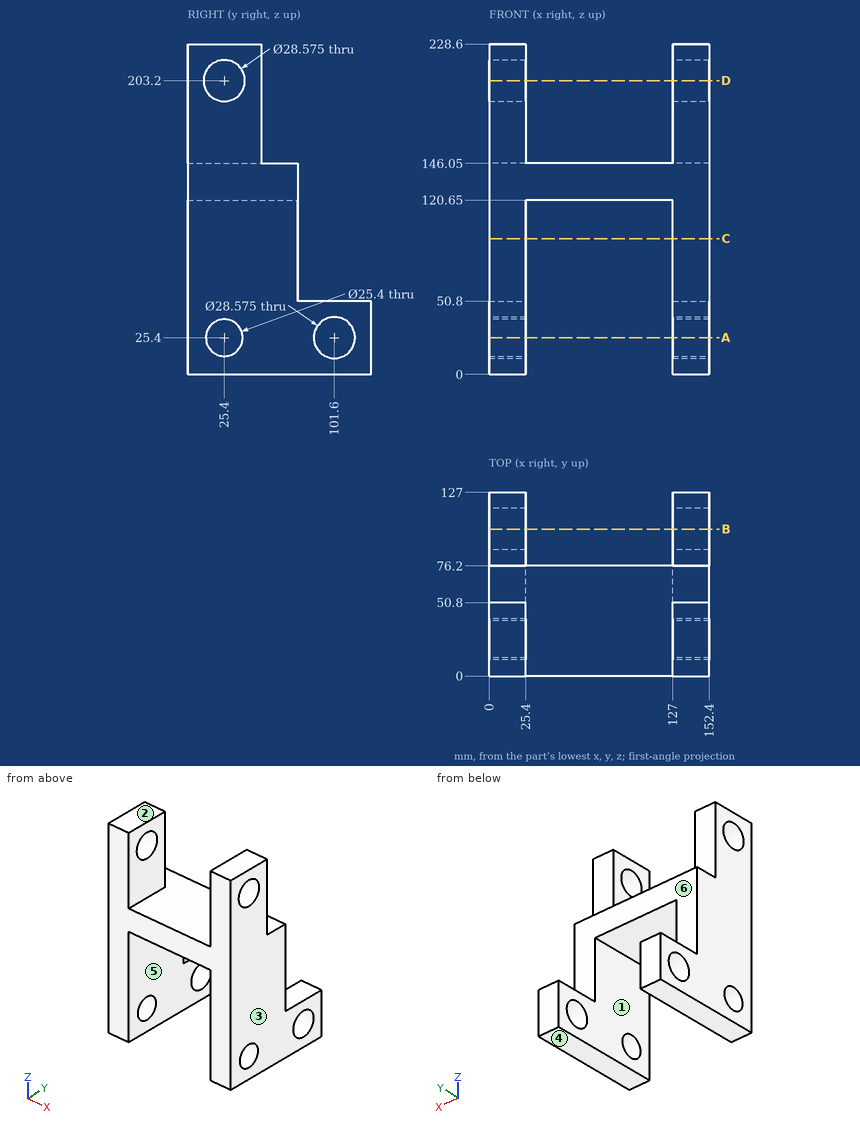
Can you work these out from the drawing? Everything is in mm from the part's minimum corner. A direction names the side the tool comes from. Give positions to 0.01 mm unless a question says otherwise; leave off trailing zeros. Write each loop counter-clockwise with the first axis right and the second up, starting at its lowest first coordinate (ties: lowest second). Pieces come first, ordered by that corner, then holes. Notation, with made-up numbers: M -2.75,-9 L 1.25,-9 A15 cw 1.25,10 Z; hole C 62.5,52 d2. An arc over 180 degrees is marked long. Answer in a Markdown table with one row per item. Add a question column.
Item 1: For pin 1 Ø2 at (x, z) = (24, 62.5) entering from +Y; pin 2 Ø2 at (x, y) = (26, 58) entering from +Z; pin 3 Ø20.5 at (x, z) = (135, 172.5) entering from +Y; pin 4 Ø10 at (x, z) = (42, 151.5) entering from -Y, each with a flat end and sliding along its axis, tell me the tip position at first contact or that it passes through.
Item 2: Imagine slicing it at B-B, the plane y = 101.6. Write out the boundary of the cut face in (x, z).
Item 3: On a 3-axis mill with a long thin cutter (end or side, diameter ignored), from which of +Z, -Z, +X, -X, +Y, -Y can I reach the whole of each face in a straight line? I mean the marked faces 4, 5 and 6. Say none if no direction works.
Item 4: Imagine slicing it at A-A, the plane z = 25.4. Write out the boundary of the cut face in (x, y).
Item 5: We'd pull the mould along X, two halves only. Please class the marked faces 1, 2 and 3: released by +X, released by -X, zero draft, split by the parting line, or undercut.
Item 6: Imagine slicing it at C-C, the plane z = 94. Write out the boundary of the cut face in (x, y), plus the area to 3 significant figures.
Item 7: Please list where these lines run through material, in increasing order: L1, parallel to Y at x = 143, z = 25; L2, parallel to X at y = 66, z = 65; L3, parallel to Z at x = 139, y = 25.
Evaluation:
| question | item | result |
|---|---|---|
| 1 | pin 1 | stops at y = 76.2 |
| 1 | pin 2 | stops at z = 146.05 |
| 1 | pin 3 | stops at y = 50.8 |
| 1 | pin 4 | passes through |
| 2 | outline | M 0,0 L 25.4,0 L 25.4,11.11 L 0,11.11 Z; M 0,39.69 L 25.4,39.69 L 25.4,50.8 L 0,50.8 Z; M 127,0 L 152.4,0 L 152.4,11.11 L 127,11.11 Z; M 127,39.69 L 152.4,39.69 L 152.4,50.8 L 127,50.8 Z |
| 3 | face 4 | -Z, +X, -X, +Y, -Y |
| 3 | face 5 | -Z, +Y, -Y |
| 3 | face 6 | +Z, +X, -X, +Y |
| 4 | outline | M 0,0 L 25.4,0 L 25.4,12.7 L 0,12.7 Z; M 0,38.1 L 25.4,38.1 L 25.4,87.31 L 0,87.31 Z; M 0,115.89 L 25.4,115.89 L 25.4,127 L 0,127 Z; M 127,0 L 152.4,0 L 152.4,12.7 L 127,12.7 Z; M 127,38.1 L 152.4,38.1 L 152.4,87.31 L 127,87.31 Z; M 127,115.89 L 152.4,115.89 L 152.4,127 L 127,127 Z |
| 5 | face 1 | undercut |
| 5 | face 2 | zero draft |
| 5 | face 3 | released by +X |
| 6 | outline | M 0,0 L 25.4,0 L 25.4,76.2 L 0,76.2 Z; M 127,0 L 152.4,0 L 152.4,76.2 L 127,76.2 Z |
| 6 | area | 3,870 mm² |
| 7 | L1 | y = 0 to 12.71, 38.09 to 87.32, 115.88 to 127 |
| 7 | L2 | x = 0 to 25.4, 127 to 152.4 |
| 7 | L3 | z = 0 to 12.71, 38.09 to 188.92, 217.48 to 228.6 |
